The listing builds one solid part. Answer for the finished solid, in the listing's coordinates (mm). Face numbers are marked on the shaded views. A direction names the side the tool comes from. Coordinates: 2 decimals unless noted, no trailing zeros. Write each loop counter-clockwise with the first axis right and the second up, starting at its lowest first coordinate (ties: lowest second). Pieces come first, ordered by that corner, then holes.
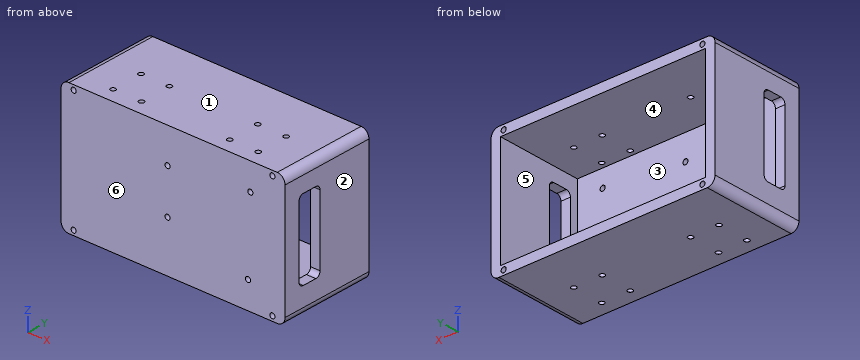
from build123d import *

# Parameters (mm, degrees)
SKETCH1_W                      = 142
SKETCH1_H                      = 82
BOSS_EXTRUDE1_DEPTH            = 60
SKETCH2_W                      = 130
SKETCH2_H                      = 70
CUT_EXTRUDE1_DEPTH             = 55
M3_CLEARANCE_HOLE1_D           = 3.2
M3_CLEARANCE_HOLE1_DEPTH       = 5
M3_CLEARANCE_HOLE1_CSINK_D     = 3.25
M3_CLEARANCE_HOLE1_CSINK_ANGLE = 90
M3_CLEARANCE_HOLE1_TIP         = 0.96137699
FILLET1_R                      = 5
SKETCH9_W                      = 50
SKETCH9_H                      = 15
CUT_EXTRUDE4_DEPTH             = 143
FILLET2_R                      = 3
M3_CLEARANCE_HOLE2_D           = 3.2
M3_CLEARANCE_HOLE2_CSINK_D     = 3.25
M3_CLEARANCE_HOLE2_CSINK_ANGLE = 90
M3_CLEARANCE_HOLE3_D           = 3.2
M3_CLEARANCE_HOLE3_CSINK_D     = 3.25
M3_CLEARANCE_HOLE3_CSINK_ANGLE = 90


with BuildPart() as part:
    # Sketch1 → Boss-Extrude1 (new body)
    with BuildSketch(Plane(origin=(0, 0, 0), x_dir=(1, 0, 0), z_dir=(0, 1, 0))):
        with Locations((71, -41)):
            Rectangle(SKETCH1_W, SKETCH1_H)
    extrude(amount=BOSS_EXTRUDE1_DEPTH)

    # Sketch2 → Cut-Extrude1 (cut)
    with BuildSketch(Plane(origin=(0, 60, 0), x_dir=(1, 0, 0), z_dir=(0, 1, 0))):
        with Locations((71, -41)):
            Rectangle(SKETCH2_W, SKETCH2_H)
    extrude(amount=-CUT_EXTRUDE1_DEPTH, mode=Mode.SUBTRACT)

    # M3 Clearance Hole1
    with Locations(Plane(origin=(0, 5, 0), x_dir=(1, 0, 0), z_dir=(0, 1, 0))):
        with Locations((118.5, -17), (120, -65), (67.5, -32), (67.5, -60)):
            CounterSinkHole(M3_CLEARANCE_HOLE1_D / 2, M3_CLEARANCE_HOLE1_CSINK_D / 2, depth=M3_CLEARANCE_HOLE1_DEPTH, counter_sink_angle=M3_CLEARANCE_HOLE1_CSINK_ANGLE)
            with Locations((0, 0, -(M3_CLEARANCE_HOLE1_DEPTH + M3_CLEARANCE_HOLE1_TIP / 2))):  # 118° drill point
                Cone(0, M3_CLEARANCE_HOLE1_D / 2, M3_CLEARANCE_HOLE1_TIP, mode=Mode.SUBTRACT)

    # Fillet1
    fillet1_edges = [part.edges().sort_by_distance(p)[0] for p in [
        (0, 30, 82),
        (0, 30, 0),
        (142, 30, 0),
        (142, 30, 82),
    ]]
    fillet(fillet1_edges, radius=FILLET1_R)

    # Sketch9 → Cut-Extrude4 (cut, through all)
    with BuildSketch(Plane(origin=(142, 0, 0), x_dir=(0, 0, -1), z_dir=(1, 0, 0))):
        with Locations((-42, 17.5)):
            Rectangle(SKETCH9_W, SKETCH9_H)
    extrude(amount=-CUT_EXTRUDE4_DEPTH, mode=Mode.SUBTRACT)

    # Fillet2
    fillet2_edges = [part.edges().sort_by_distance(p)[0] for p in [
        (139, 10, 17),
        (139, 10, 67),
        (139, 25, 67),
        (139, 25, 17),
        (3, 10, 17),
        (3, 10, 67),
        (3, 25, 67),
        (3, 25, 17),
    ]]
    fillet(fillet2_edges, radius=FILLET2_R)

    # M3 Clearance Hole2 (through all)
    with Locations(Plane(origin=(0, 60, 0), x_dir=(1, 0, 0), z_dir=(0, 1, 0))):
        with Locations((8, -3), (8, -79), (134, -79), (134, -3)):
            CounterSinkHole(M3_CLEARANCE_HOLE2_D / 2, M3_CLEARANCE_HOLE2_CSINK_D / 2, counter_sink_angle=M3_CLEARANCE_HOLE2_CSINK_ANGLE)

    # M3 Clearance Hole3 (through all)
    with Locations(Plane(origin=(0, 0, 0), x_dir=(-1, 0, 0), z_dir=(0, 0, -1))):
        with Locations((-117, 29), (-99, 29), (-117, 9), (-99, 9), (-25, 9), (-43, 9), (-43, 29), (-25, 29)):
            CounterSinkHole(M3_CLEARANCE_HOLE3_D / 2, M3_CLEARANCE_HOLE3_CSINK_D / 2, counter_sink_angle=M3_CLEARANCE_HOLE3_CSINK_ANGLE)


solid = part.part
1. Section D-D on x = 67.5 is taken. Give the vertices of the cut face in (y, z) (3 decimals), then the cut area to 3 significant figures.
Results found:
outline: (0, 0) - (60, 0) - (60, 6) - (5, 6) - (5, 30.375) - (4.975, 30.4) - (0, 30.4) - close; (0, 33.6) - (4.975, 33.6) - (5, 33.625) - (5, 58.375) - (4.975, 58.4) - (0, 58.4) - close; (0, 61.6) - (4.975, 61.6) - (5, 61.625) - (5, 76) - (60, 76) - (60, 82) - (0, 82) - close
area: 1,040 mm2
2. A tool of negligible diameter and unlimited length cuts with its end or side. For the marked faces 5 and 6, from which of +Z, -Z, +X, -X, +Y, -Y can it reach the whole face along a straight path? Write none if from no direction.
Results found:
face 5: +Y
face 6: +Z, -Z, +X, -X, -Y
3. Find the intervals of material crossed by L1, parallel to Z at x = 47, y = 57; L2, parallel to X at y = 28.5, z = 35.5; L3, parallel to Z at x = 9, y = 25, in increasing order.
Results found:
L1: z = 0 to 6, 76 to 82
L2: x = 0 to 6, 136 to 142
L3: z = 0 to 1.75, 4.25 to 6, 76 to 77.75, 80.25 to 82
4. Section C-C on y = 36 is taken. Give the vertices of the cut face in (x, z).
Results found:
outline: (0, 5) arc R5 ccw to (5, 0) - (137, 0) arc R5 ccw to (142, 5) - (142, 77) arc R5 ccw to (137, 82) - (5, 82) arc R5 ccw to (0, 77) - close; hole (6, 6) - (136, 6) - (136, 76) - (6, 76) - close; hole circle Ø3.2 at (8, 3); hole circle Ø3.2 at (8, 79); hole circle Ø3.2 at (134, 3); hole circle Ø3.2 at (134, 79)
5. Section A-A on z = 39 is taken. Give the vertices of the cut face in (x, y), then the cut area to 3 significant figures.
Results found:
outline: (0, 0) - (142, 0) - (142, 10) - (136, 10) - (136, 5) - (6, 5) - (6, 10) - (0, 10) - close; (0, 25) - (6, 25) - (6, 60) - (0, 60) - close; (136, 25) - (142, 25) - (142, 60) - (136, 60) - close
area: 1,190 mm2
6. A flat-ended cylindrical pin translates along its axis: P1, Ø1, axis at x = 46.5, z = 13, coming from the +Y side. Find the tip coordinate at first contact, or state that the pin passes through.
Results found:
P1: stops at y = 5
7. For a pull along X with two mould halves and no side action, classify the marked faces 1, 2, 3 and 4 as pulls with the +X half, pulls with the -X half, needs draft (parallel to the pull), parting line crosses it, or undercut.
Results found:
face 1: needs draft
face 2: pulls with the +X half
face 3: undercut
face 4: undercut
8. Section B-B on x = 43 is taken. Give the vertices of the cut face in (y, z) (3 decimals).
Results found:
outline: (0, 0) - (7.375, 0) - (7.4, 0.025) - (7.4, 6) - (5, 6) - (5, 76) - (7.4, 76) - (7.4, 82) - (0, 82) - close; (10.6, 0.025) - (10.625, 0) - (27.375, 0) - (27.4, 0.025) - (27.4, 6) - (10.6, 6) - close; (10.6, 76) - (27.4, 76) - (27.4, 82) - (10.6, 82) - close; (30.6, 0.025) - (30.625, 0) - (60, 0) - (60, 6) - (30.6, 6) - close; (30.6, 76) - (60, 76) - (60, 82) - (30.6, 82) - close
